Verification items for the finished model (mm, model axes). Face numbers are marked on the shaded views. A direction names the side the tool comes from. Give positions to 0.01 mm unless a question says otherwise; leave off trailing zeros. Order: outer loops, then holes, each group sorted by start corner. A loop starts at its lowest first (then second) coordinate and runs counter-clockwise, first axis right, second up. Notation, with made-up numbers: (-27, 81) -> (2, 81) arc R28 ccw to (2, 107) -> close; hole circle Ø1 at (-3, -10). An arc over 180 degrees is marked (long way). Return JSON: item names as keys, results as strings. Group by question number.
(1) Depth check by flat-ended pin: pin 1 Ø3 at (x, y) = (4, 1) entering from +Z. Enter the tip coordinate at first touch or a pass-through.
(2) Release check for a two-part mould opening along X. For the marked faces 3, 4, 5 and 6 record: pulls with the +X half, pulls with the -X half, needs draft (parallel to the pull), parting line crosses it, or undercut.
(3) Cross-section at B-B on y = 2. Enter the section's corners in (x, z) (3 decimals).
(4) Cross-section at D-D on z = 1.5. Enter the section's corners in (x, y).
(5) Tool access check on the marked faces 1 and 2. Record the directions out of +Z, -Z, +X, -X, +Y, -Y that give a thin tool (end or side, any length) a straight path to the whole face; none if there is none.
(6) Cross-section at C-C on x = -2.31. Enter the section's corners in (y, z), then the cut area to 3 significant figures.
(7) Thickness scan on line 1 along X through (y, z) = (-1.5, 2.25); line 2 along Z through (x, y) = (4.69, 1.75) (3 decimals); line 3 along X through (y, z) = (0.75, 8.4). Record the ranges inside material, lowest first.
(8) Cross-section at A-A on x = 4.69. Enter the section's corners in (y, z) (3 decimals), then the cut area to 3 significant figures.
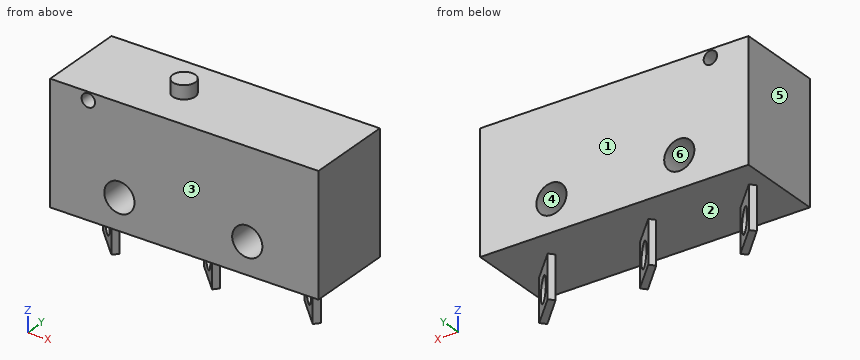
from build123d import *

# Parameters (mm, degrees)
SKETCH_1_W             = 20
SKETCH_1_H             = 6.5
EXTRUDE_1_DEPTH        = 9
HOLE_WIZARD_1_D        = 2.25
SKETCH_7_R             = 0.838393999
EXTRUDE_2_DEPTH        = 1
HOLE_WIZARD_2_D        = 1
EXTRUDE_3_DEPTH        = 3.2
HOLE_WIZARD_3_D        = 1.8
HOLE_WIZARD_3_DEPTH    = 6.5
PATTERN_LINEAR_1_COUNT = 3
PATTERN_LINEAR_1_PITCH = 7.5


with BuildPart() as part:
    # ｽｹｯﾁ1 → ﾎﾞｽ - 押し出し1 (new body)
    with BuildSketch(Plane.XY):
        Rectangle(SKETCH_1_W, SKETCH_1_H)
    extrude(amount=EXTRUDE_1_DEPTH)

    # 穴1 (through all)
    with Locations(Plane(origin=(0, -3.25, 0), x_dir=(-1, 0, 0), z_dir=(0, -1, 0))):
        with Locations((4.84, -2.35), (-4.69, -2.35)):
            Hole(HOLE_WIZARD_1_D / 2)

    # ｽｹｯﾁ7 → ﾎﾞｽ - 押し出し2 (add)
    with BuildSketch(Plane.XY.offset(9)):
        with Locations(Location((-2.31, 0, 0), (0, 0, 180))):
            Circle(SKETCH_7_R)
    extrude(amount=EXTRUDE_2_DEPTH)

    # 穴2 (through all)
    with Locations(Plane(origin=(0, -3.25, 0), x_dir=(-1, 0, 0), z_dir=(0, -1, 0))):
        with Locations((7.16, -8.4)):
            Hole(HOLE_WIZARD_2_D / 2)

    # ｽｹｯﾁ10 → ﾎﾞｽ - 押し出し3 (add)
    with BuildSketch(Plane(origin=(0, 0, 0), x_dir=(-1, 0, 0), z_dir=(0, 0, -1))):
        Polygon((-6.381555021, 1.244871931), (-8.509905901, -0.883478949), (-8.172897935, -1.265123133), (-6.058582994, 0.863179555), align=None)
    extrude_3 = extrude(amount=EXTRUDE_3_DEPTH)

    # 穴3
    with Locations(Plane(origin=(3.813213476, 3.813213476, 0), x_dir=(0, 0, -1), z_dir=(0.7071067811865488, 0.7071067811865462, 0))):
        with Locations((1.7, -5.132183446)):
            hole_wizard_3 = Hole(HOLE_WIZARD_3_D / 2, depth=HOLE_WIZARD_3_DEPTH)

    # 直線ﾊﾟﾀｰﾝ1: ﾎﾞｽ - 押し出し3, 穴3 ×3
    with Locations(*[(-i * PATTERN_LINEAR_1_PITCH, 0, 0) for i in range(1, PATTERN_LINEAR_1_COUNT)]):
        add(extrude_3)
        add(hole_wizard_3, mode=Mode.SUBTRACT)


solid = part.part
Verdict:
{
 "1": {"pin 1": "z = 9"},
 "2": {"face 3": "needs draft", "face 4": "undercut", "face 5": "pulls with the -X half", "face 6": "undercut"},
 "3": {"outline": "(-10, 0) -> (10, 0) -> (10, 9) -> (-10, 9) -> close; hole circle Ø1 at (-7.16, 8.4); hole circle Ø2.25 at (-4.84, 2.35); hole circle Ø2.25 at (4.69, 2.35)"},
 "4": {"outline": "(-10, -3.25) -> (-5.58, -3.25) -> (-5.58, 3.25) -> (-10, 3.25) -> close; (-4.1, -3.25) -> (3.95, -3.25) -> (3.95, 3.25) -> (-4.1, 3.25) -> close; (5.43, -3.25) -> (10, -3.25) -> (10, 3.25) -> (5.43, 3.25) -> close"},
 "5": {"face 1": "+Z, -Z, +X, -X, +Y", "face 2": "-Z"},
 "6": {"outline": "(-3.25, 0) -> (3.25, 0) -> (3.25, 9) -> (0.84, 9) -> (0.84, 10) -> (-0.84, 10) -> (-0.84, 9) -> (-3.25, 9) -> close", "area": "60.2 mm²"},
 "7": {"line 1": "-10 to -5.96, -3.72 to 3.57, 5.81 to 10", "line 2": "0 to 1.225, 3.475 to 9", "line 3": "-10 to -7.66, -6.66 to 10"},
 "8": {"outline": "(-3.25, 0) -> (3.25, 0) -> (3.25, 1.225) -> (-3.25, 1.225) -> close; (-3.25, 3.475) -> (3.25, 3.475) -> (3.25, 9) -> (-3.25, 9) -> close", "area": "43.9 mm²"}
}
